Check sheet for the modelled part. Datum: model origin and axes. Units: mm. Face numbers are marked on the shaded views. A direction names the side the tool comes from. Give positions to 0.01 mm unless a question says otherwise; leave off trailing zeros. Write each loop counter-clockwise with the first axis right and the second up, starting at its lowest first coordinate (ties: lowest second). Pieces come first, ordered by that corner, then holes. Notation, with made-up numbers: (88, 57) -> (125, 57) arc R20 cw to (125, 80) -> close; hole circle Ø8 at (31.5, 14.25). An arc over 180 degrees is marked (long way). Answer as a JSON object with one key per item and string values.
from build123d import *


with BuildPart() as f1:
    # F0 (on Top) → F1 (revolve)
    with BuildSketch(Plane.XY):
        with BuildLine():
            Line((-10.863817, 4.514776), (-14.713817, 4.514776))
            Line((-14.713817, 4.514776), (-14.713817, 2.514776))
            ThreePointArc((-14.713817, 2.514776), (-13.398503, 2.029725), (-12.447191, 1))
            Line((-12.447191, 1), (-1.843817, 1))
            Line((-1.843817, 1), (-1.843817, 1.879776))
            Line((-1.843817, 1.879776), (-10.863817, 3.014776))
            Line((-10.863817, 3.014776), (-10.863817, 4.514776))
        make_face()
    revolve(axis=Axis((-25.231563, 0, 0), (1, 0, 0)))


solid = f1.part
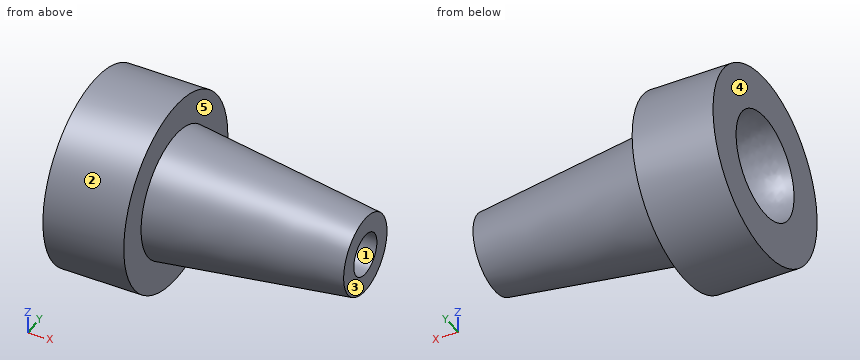
1. Sectioned sample at A-A, the plane x = -11.75. Enter the section's corners in (y, z), plus the area to 3 significant figures.
Determined:
{"outline": "circle Ø9.03 at (0, 0); hole circle Ø2 at (0, 0)", "area": "60.9 mm^2"}
2. Sectioned sample at B-B, the plane z = 4.25. Enter the section's corners in (x, y), plus the area to 3 significant figures.
Determined:
{"outline": "(-14.71, -1.52) -> (-10.86, -1.52) -> (-10.86, 1.52) -> (-14.71, 1.52) -> close", "area": "11.7 mm^2"}
3. Sectioned sample at C-C, the plane x = -3.75. Enter the section's corners in (y, z), plus the area to 3 significant figures.
Determined:
{"outline": "circle Ø4.24 at (0, 0); hole circle Ø2 at (0, 0)", "area": "11.0 mm^2"}
4. Scan lines: L1, parallel to X at y = 0.75, z = 3.5; L2, parallel to Z at x = -6, y = -0.5; L3, parallel to Z at x = -4.5, y = -0.25. Record each from-to range of solid material in increasing order. Write a range as [from, to].
Determined:
{"L1": "[-14.71, -10.86]", "L2": "[-2.35, -0.87], [0.87, 2.35]", "L3": "[-2.2, -0.97], [0.97, 2.2]"}
5. Access from +Z, -Z, +X, -X, +Y, -Y to the whole of each face (thin tool, end or side, straight path). Record for the marked faces 4 and 5.
Determined:
{"face 4": "+Z, -Z, -X, +Y, -Y", "face 5": "+X"}
6. Mould release check, pull along Z, two halves, no side actions. Record for the marked faces 1, 2 and 3: released by +Z, released by -Z, zero draft, split by the parting line, or undercut.
Determined:
{"face 1": "undercut", "face 2": "split by the parting line", "face 3": "zero draft"}
7. Go/stop test with flat-tipped pins: P1, Ø1.8, axis at y = 0, z = 0, coming from the -X side; P2, Ø1, axis at y = -1.5, z = 1, coming from the -X side; P3, Ø1, axis at x = -12.5, y = -2.5, coming from the +Z side; P4, Ø3, axis at x = -3.5, z = 3, coming from the -Y side. Record where each tip stops, or that it passes through.
Determined:
{"P1": "through", "P2": "x = -13.91", "P3": "z = 4.05", "P4": "y = -1.48"}
